from build123d import *
from build123d.topology import SkipClean

# Parameters (mm, degrees)
SKETCH2_R            = 8
BOSS_EXTRUDE1_DEPTH  = 9.25
SKETCH3_R            = 8
BOSS_EXTRUDE2_DEPTH  = 9.25
SKETCH5_R            = 22.5
BOSS_EXTRUDE3_DEPTH  = 20
SKETCH6_R            = 9.5
CUT_EXTRUDE1_DEPTH   = 20
CUT_EXTRUDE3_DEPTH   = 9.5
FILLET1_R            = 7.5
FILLET1_OF_MIRROR1_R = 7.5
SKETCH9_R            = 22.5
SKETCH9_R_2          = 9.5
BOSS_EXTRUDE5_DEPTH  = 6.35


with BuildPart() as part:
    # Sketch2 → Boss-Extrude1 (new, symmetric)
    with BuildSketch(Plane(origin=(0, 0, 0), x_dir=(1, 0, 0), z_dir=(0, 1, 0))):
        with BuildLine():
            Line((0, -20), (-120, -20))
            ThreePointArc((-120, -20), (-140, 0), (-120, 20))
            Line((-120, 20), (0, 20))
            Line((0, 20), (0, -20))
        make_face()
        with Locations(Location((-120, 0, 0), (0, 0, 270))):
            Circle(SKETCH2_R, mode=Mode.SUBTRACT)
    extrude(amount=BOSS_EXTRUDE1_DEPTH, both=True)

    # Sketch3 → Boss-Extrude2 (add, symmetric)
    with BuildSketch(Plane(origin=(0, 0, 0), x_dir=(0.5735764363510444, -0.819152044288993, 0), z_dir=(0.819152044288993, 0.5735764363510444, 0))):
        with BuildLine():
            Line((0, -20), (-127.5, -20))
            ThreePointArc((-127.5, -20), (-147.5, 0), (-127.5, 20))
            Line((-127.5, 20), (0, 20))
            Line((0, 20), (0, -20))
        make_face()
        with Locations(Location((-127.5, 0, 0), (0, 0, 180))):
            Circle(SKETCH3_R, mode=Mode.SUBTRACT)
    extrude(amount=BOSS_EXTRUDE2_DEPTH, both=True)

    # Sketch5 → Boss-Extrude3 (add, symmetric)
    with BuildSketch(Plane.XY):
        with BuildLine():
            Line((-88.25, -22.5), (0, -22.5))
            ThreePointArc((0, -22.5), (-19.957743747, 10.389343798), (18.430920997, 12.905469818))
            Line((18.430920997, 12.905469818), (-31.393139414, 84.061602381))
            Line((-31.393139414, 84.061602381), (-88.25, 44.25))
            Line((-88.25, 44.25), (-88.25, -22.5))
        make_face()
        Circle(SKETCH5_R)
    extrude(amount=BOSS_EXTRUDE3_DEPTH, both=True)

    # Sketch6 → Cut-Extrude1 (cut, symmetric)
    with BuildSketch(Plane.XY):
        Circle(SKETCH6_R)
    extrude(amount=CUT_EXTRUDE1_DEPTH, both=True, mode=Mode.SUBTRACT)

    # Sketch7 → Cut-Extrude3 (cut)
    with BuildSketch(Plane.XY.offset(20)):
        with BuildLine():
            Line((-78.75, -22.5), (0, -22.5))
            ThreePointArc((0, -22.5), (-12.093386622, -18.973665961), (-20.396078054, -9.5))
            Line((-20.396078054, -9.5), (-78.75, -9.5))
            Line((-78.75, -9.5), (-78.75, -22.5))
        make_face()
        with BuildLine():
            Line((-25.944163269, 76.27965796), (-36.797927856, 68.679770179))
            Line((-36.797927856, 68.679770179), (-4.187279424, 22.106937622))
            ThreePointArc((-4.187279424, 22.106937622), (8.47862511, 20.841375105), (18.430920997, 12.905469818))
            Line((18.430920997, 12.905469818), (-25.944163269, 76.27965796))
        make_face()
        Polygon((-17.944136559, 9.5), (-51.952240675, 58.068606106), (-78.75, 39.30461302), (-78.75, 9.5), align=None)
    cut_extrude3 = extrude(amount=-CUT_EXTRUDE3_DEPTH, mode=Mode.SUBTRACT)

    # Fillet1
    fillet1_edges = [part.edges().sort_by_distance(p)[0] for p in [
        (-20.396078054, -9.5, 15.25),
        (-78.75, -9.5, 15.25),
        (-78.75, 39.30461302, 15.25),
        (-51.952240675, 58.068606106, 15.25),
        (-17.944136559, 9.5, 15.25),
        (-78.75, 9.5, 15.25),
        (-4.187279424, 22.106937622, 15.25),
        (-36.797927856, 68.679770179, 15.25),
    ]]
    fillet(fillet1_edges, radius=FILLET1_R)

    # Mirror1: Cut-Extrude3 across plane
    add(cut_extrude3.mirror(Plane.XY), mode=Mode.SUBTRACT)

    # Fillet1 of Mirror1
    fillet1_of_mirror1_edges = [part.edges().sort_by_distance(p)[0] for p in [
        (-20.396078054, -9.5, -15.25),
        (-78.75, -9.5, -15.25),
        (-78.75, 39.30461302, -15.25),
        (-51.952240675, 58.068606106, -15.25),
        (-17.944136559, 9.5, -15.25),
        (-78.75, 9.5, -15.25),
        (-4.187279424, 22.106937622, -15.25),
        (-36.797927856, 68.679770179, -15.25),
    ]]
    fillet(fillet1_of_mirror1_edges, radius=FILLET1_OF_MIRROR1_R)

    # Sketch9 → Boss-Extrude5 (add)
    with SkipClean():  # the faces are left unmerged after this step: merging them gives an invalid solid
        with BuildSketch(Plane.XY.offset(20)):
            with Locations(Location((0, 0, 0), (0, 0, 214.518107841))):
                Circle(SKETCH9_R)
            Circle(SKETCH9_R_2, mode=Mode.SUBTRACT)
        boss_extrude5 = extrude(amount=BOSS_EXTRUDE5_DEPTH)

    # Mirror2: Boss-Extrude5 across plane
    with SkipClean():  # the faces are left unmerged after this step: merging them gives an invalid solid
        add(boss_extrude5.mirror(Plane.XY))


solid = part.part
Geometry check sheet. Reference: the model listing, model coordinates, mm. A direction names the side the tool comes from. Give positions to 0.01 mm unless a question says otherwise; leave off trailing zeros. Order: outer loops, then holes, each group sorted by start corner. A loop starts at its lowest first (then second) coordinate and runs counter-clockwise, first axis right, second up.
1. Sectioned sample at A-A (y = 0). Record the boundary of the cut face in (x, z), then the cut area to 3 significant figures.
Completed:
outline: (-120, -20) - (-22.5, -20) - (-22.5, -26.35) - (-9.5, -26.35) - (-9.5, 26.35) - (-22.5, 26.35) - (-22.5, 20) - (-120, 20) arc R20 ccw to start; (9.5, -26.35) - (22.5, -26.35) - (22.5, 26.35) - (9.5, 26.35) - close; hole circle Ø16 at (-120, 0)
area: 5,700 mm2
2. Access from +Z, -Z, +X, -X, +Y, -Y to the whole of each face (thin tool, end or side, straight path). Record for faces 1 (the face through (-52, 28, 10.5)), 2 (the face through (-12, 47, 10.5)), 3 (the face through (-77.88, 38.91, -15.18)), 4 (the face through (-76.611, -11.755, 15.183)).
Completed:
face 1: +Z
face 2: +Z, +X
face 3: -Z
face 4: +Z, -Y
3. Sectioned sample at C-C (x = 6). Record the boundary of the cut face in (y, z).
Completed:
outline: (-21.69, -26.35) - (-7.37, -26.35) - (-7.37, 26.35) - (-21.69, 26.35) - close; (7.37, -26.35) - (21.69, -26.35) - (21.69, -10.5) - (30.66, -10.5) - (30.66, 10.5) - (21.69, 10.5) - (21.69, 26.35) - (7.37, 26.35) - close
4. Sectioned sample at B-B (z = 0). Record the boundary of the cut face in (x, y), then the cut area to 3 significant figures.
Completed:
outline: (-140, -9.25) - (-128, -9.25) - (-128, 9.25) - (-140, 9.25) - close; (-112, -9.25) - (-88.25, -9.25) - (-88.25, -22.5) - (0, -22.5) arc R22.5 ccw to (18.43, 12.91) - (-31.39, 84.06) - (-42.25, 76.46) - (-60.97, 103.19) - (-76.12, 92.58) - (-57.4, 65.85) - (-88.25, 44.25) - (-88.25, 9.25) - (-112, 9.25) - close; (-92.18, 115.52) - (-85.3, 105.69) - (-70.14, 116.3) - (-77.03, 126.13) - close; hole circle Ø19 at (0, 0)
area: 9,690 mm2
5. Sectioned sample at D-D (z = 22.5). Record the boundary of the cut face in (x, y).
Completed:
outline: circle Ø45 at (0, 0); hole circle Ø19 at (0, 0)
6. Depth check by flat-ended pin: pin 1 (6 mm diameter, centred on y = 66, z = -9, fed in from -X); pin 2 (1.6 mm diameter, centred on y = -19, z = -13, fed in from +X); pin 3 (5 mm diameter, centred on x = -53.5, z = -17, fed in from -Y). Enter the tip coordinate at first touch or a pass-through.
Completed:
pin 1: stops at x = -61.47
pin 2: stops at x = 13.23
pin 3: stops at y = -9.5
7. Scan lines: line 1 (Y direction, x = 0, z = 21.5); line 2 (Y direction, x = -70, z = -11); line 3 (Y direction, x = -62, z = 16). Record each from-to range of solid material in increasing order.
Completed:
line 1: y = -22.5 to -9.5, 9.5 to 22.5
line 2: y = -9.5 to 9.5, 45.43 to 57.03, 83.84 to 116.1
line 3: y = -9.5 to 9.5, 51.03 to 62.63, 72.42 to 104.67
8. Draft check along X on faces 5 (the face through (-48, -9.5, -15)), 6 (the face through (-72.61, 55.2, 0.28)), 7 (the face through (-74, 44, -20)). Enter one of: pulls with the +X half, pulls with the -X half, needs draft (parallel to the pull), parting line crosses it, or undercut.
Completed:
face 5: undercut
face 6: pulls with the -X half
face 7: needs draft
